Verification items for this drawing (mm, ordinates from the low corner). A direction names the side the tool comes from. Coordinates: 2 decimals unless noted, no trailing zeros. Order: outer loops, then holes, each group sorted by start corner. A loop starts at its lowest first (then second) coordinate and runs counter-clockwise, first axis right, second up. Notation, with made-up numbers: (69, -29) -> (117, -29) arc R15 cw to (117, -7) -> close; hole circle Ø1 at (35.25, 57.25). An arc over 180 degrees is marked (long way). Write item = value, one per line. Start each with the question number.
1. Set-up check for the marked faces 4, 5, 6, 7 and 8: record each of +Z, -Z, +X, -X, +Y, -Y from which the full face is reachable in a straight line by a thin tool's end or side.
2. Cross-section at C-C on y = 9.25. Record the cut outline in (x, z).
3. Release check for a two-part mould opening along X. For the marked faces 1, 2 and 3 record: +X half, -X half, draft (parallel to the pull), parting line (faces both ways), or undercut.
4. Thickness scan on line 1 along Z through (x, y) = (8.75, 7.5); line 2 along Y through (x, z) = (6, 1.8); line 3 along Y through (x, z) = (6.5, 1.5). Record the ranges inside material, lowest first. Write a range as from..to.
5. Go/stop test with flat-tipped pins: P1, Ø3, axis at x = 2.5, y = 7, coming from the -Z side; P2, Ø1, axis at x = 6.5, z = 4, coming from the +Y side; P3, Ø5, axis at x = 4.5, y = 6, coming from the +Z side. Record where each tip stops, or that it passes through.
6. Cross-section at D-D on z = 1.75. Record the cut outline in (x, y), plus the area to 3 significant figures.
7. Cross-section at A-A on y = 6.5. Record the cut outline in (x, z), plus the area to 3 significant figures.
8. Cross-section at B-B on x = 6. Give the number of separate pieces and of enclosed holes in the cut face.
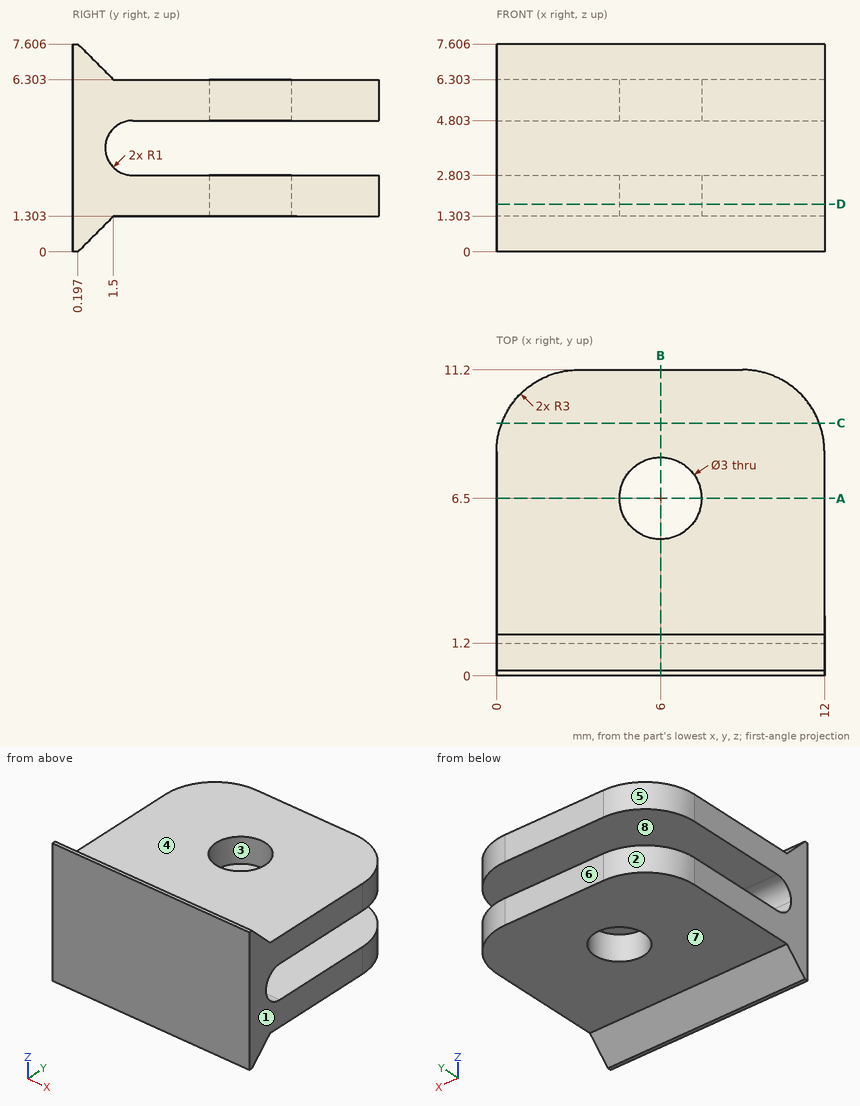
Worked out:
q1.face_4 = +Z, +X, -X, +Y
q1.face_5 = +Z, -Z, -X, +Y
q1.face_6 = +Z, -Z, +X, -X, +Y
q1.face_7 = -Z, +X, -X, +Y
q1.face_8 = +X, -X, +Y
q2.outline = (0.19, 1.3) -> (11.81, 1.3) -> (11.81, 2.8) -> (0.19, 2.8) -> close; (0.19, 4.8) -> (11.81, 4.8) -> (11.81, 6.3) -> (0.19, 6.3) -> close
q3.face_1 = +X half
q3.face_2 = -X half
q3.face_3 = undercut
q4.line_1 = 1.3..2.8, 4.8..6.3
q4.line_2 = 0..5, 8..11.2
q4.line_3 = 0..5.09, 7.91..11.2
q5.P1 = 1.3
q5.P2 = 1.48
q5.P3 = 6.3
q6.outline = (0, 0) -> (12, 0) -> (12, 8.2) arc R3 ccw to (9, 11.2) -> (3, 11.2) arc R3 ccw to (0, 8.2) -> close; hole circle Ø3 at (6, 6.5)
q6.area = 123 mm²
q7.outline = (0, 1.3) -> (4.5, 1.3) -> (4.5, 2.8) -> (0, 2.8) -> close; (0, 4.8) -> (4.5, 4.8) -> (4.5, 6.3) -> (0, 6.3) -> close; (7.5, 1.3) -> (12, 1.3) -> (12, 2.8) -> (7.5, 2.8) -> close; (7.5, 4.8) -> (12, 4.8) -> (12, 6.3) -> (7.5, 6.3) -> close
q7.area = 27.0 mm²
q8.separate_pieces = 3
q8.enclosed_holes = 0
